```python
from build123d import *

# Parameters (mm, degrees)
F0_R     = 2.5
F1_DEPTH = 25


with BuildPart() as f1:
    # F0 (on Top) → F1 (new body)
    with BuildSketch(Plane.XY):
        with BuildLine():
            Line((-0.206975, 3.902523), (-2.845819, 3.902523))
            Line((-2.845819, 3.902523), (-5.497237, 6.55394))
            Line((-5.497237, 6.55394), (-5.497237, 8.202523))
            Line((-5.497237, 8.202523), (-2.885113, 8.202523))
            Line((-2.885113, 8.202523), (-2.885113, 8.30915))
            Line((-2.885113, 8.30915), (-4.400227, 9.824264))
            ThreePointArc((-4.400227, 9.824264), (-4.594881, 9.954328), (-4.824491, 10))
            Line((-4.824491, 10), (-8.5, 10))
            ThreePointArc((-8.5, 10), (-9.074025, 9.885819), (-9.56066, 9.56066))
            ThreePointArc((-9.56066, 9.56066), (-9.885819, 9.074025), (-10, 8.5))
            Line((-10, 8.5), (-10, 4.824491))
            ThreePointArc((-10, 4.824491), (-9.954328, 4.594881), (-9.824264, 4.400227))
            Line((-9.824264, 4.400227), (-8.30915, 2.885113))
            Line((-8.30915, 2.885113), (-8.202523, 2.885113))
            Line((-8.202523, 2.885113), (-8.202523, 5.497237))
            Line((-8.202523, 5.497237), (-6.55394, 5.497237))
            Line((-6.55394, 5.497237), (-3.902523, 2.845819))
            Line((-3.902523, 2.845819), (-3.902523, 0.206975))
            Line((-3.902523, 0.206975), (-3.695548, 0))
            Line((-3.695548, 0), (-3.902523, -0.206975))
            Line((-3.902523, -0.206975), (-3.902523, -2.845819))
            Line((-3.902523, -2.845819), (-6.55394, -5.497237))
            Line((-6.55394, -5.497237), (-8.202523, -5.497237))
            Line((-8.202523, -5.497237), (-8.202523, -2.885113))
            Line((-8.202523, -2.885113), (-8.30915, -2.885113))
            Line((-8.30915, -2.885113), (-9.824264, -4.400227))
            ThreePointArc((-9.824264, -4.400227), (-9.954328, -4.594881), (-10, -4.824491))
            Line((-10, -4.824491), (-10, -8.5))
            ThreePointArc((-10, -8.5), (-9.885819, -9.074025), (-9.56066, -9.56066))
            ThreePointArc((-9.56066, -9.56066), (-9.074025, -9.885819), (-8.5, -10))
            Line((-8.5, -10), (-4.824491, -10))
            ThreePointArc((-4.824491, -10), (-4.594881, -9.954328), (-4.400227, -9.824264))
            Line((-4.400227, -9.824264), (-2.885113, -8.30915))
            Line((-2.885113, -8.30915), (-2.885113, -8.202523))
            Line((-2.885113, -8.202523), (-5.497237, -8.202523))
            Line((-5.497237, -8.202523), (-5.497237, -6.55394))
            Line((-5.497237, -6.55394), (-2.845819, -3.902523))
            Line((-2.845819, -3.902523), (-0.206975, -3.902523))
            Line((-0.206975, -3.902523), (0, -3.695548))
            Line((0, -3.695548), (0.206975, -3.902523))
            Line((0.206975, -3.902523), (2.845819, -3.902523))
            Line((2.845819, -3.902523), (5.497237, -6.55394))
            Line((5.497237, -6.55394), (5.497237, -8.202523))
            Line((5.497237, -8.202523), (2.885113, -8.202523))
            Line((2.885113, -8.202523), (2.885113, -8.30915))
            Line((2.885113, -8.30915), (4.400227, -9.824264))
            ThreePointArc((4.400227, -9.824264), (4.594881, -9.954328), (4.824491, -10))
            Line((4.824491, -10), (8.5, -10))
            ThreePointArc((8.5, -10), (9.074025, -9.885819), (9.56066, -9.56066))
            ThreePointArc((9.56066, -9.56066), (9.885819, -9.074025), (10, -8.5))
            Line((10, -8.5), (10, -4.824491))
            ThreePointArc((10, -4.824491), (9.954328, -4.594881), (9.824264, -4.400227))
            Line((9.824264, -4.400227), (8.30915, -2.885113))
            Line((8.30915, -2.885113), (8.202523, -2.885113))
            Line((8.202523, -2.885113), (8.202523, -5.497237))
            Line((8.202523, -5.497237), (6.55394, -5.497237))
            Line((6.55394, -5.497237), (3.902523, -2.845819))
            Line((3.902523, -2.845819), (3.902523, -0.206975))
            Line((3.902523, -0.206975), (3.695548, 0))
            Line((3.695548, 0), (3.902523, 0.206975))
            Line((3.902523, 0.206975), (3.902523, 2.845819))
            Line((3.902523, 2.845819), (6.55394, 5.497237))
            Line((6.55394, 5.497237), (8.202523, 5.497237))
            Line((8.202523, 5.497237), (8.202523, 2.885113))
            Line((8.202523, 2.885113), (8.30915, 2.885113))
            Line((8.30915, 2.885113), (9.824264, 4.400227))
            ThreePointArc((9.824264, 4.400227), (9.954328, 4.594881), (10, 4.824491))
            Line((10, 4.824491), (10, 8.5))
            ThreePointArc((10, 8.5), (9.885819, 9.074025), (9.56066, 9.56066))
            ThreePointArc((9.56066, 9.56066), (9.074025, 9.885819), (8.5, 10))
            Line((8.5, 10), (4.824491, 10))
            ThreePointArc((4.824491, 10), (4.594881, 9.954328), (4.400227, 9.824264))
            Line((4.400227, 9.824264), (2.885113, 8.30915))
            Line((2.885113, 8.30915), (2.885113, 8.202523))
            Line((2.885113, 8.202523), (5.497237, 8.202523))
            Line((5.497237, 8.202523), (5.497237, 6.55394))
            Line((5.497237, 6.55394), (2.845819, 3.902523))
            Line((2.845819, 3.902523), (0.206975, 3.902523))
            Line((0.206975, 3.902523), (0, 3.695548))
            Line((0, 3.695548), (-0.206975, 3.902523))
        make_face()
        Polygon((-7.11684, -7.11684), (-6.573574, -7.660106), (-6.573574, -8.202523), (-8.202523, -8.202523), (-8.202523, -6.573574), (-7.660106, -6.573574), align=None, mode=Mode.SUBTRACT)
        Polygon((7.11684, -7.11684), (7.660106, -6.573574), (8.202523, -6.573574), (8.202523, -8.202523), (6.573574, -8.202523), (6.573574, -7.660106), align=None, mode=Mode.SUBTRACT)
        Polygon((-6.573574, 8.202523), (-6.573574, 7.660106), (-7.11684, 7.11684), (-7.660106, 6.573574), (-8.202523, 6.573574), (-8.202523, 8.202523), align=None, mode=Mode.SUBTRACT)
        Circle(F0_R, mode=Mode.SUBTRACT)
        Polygon((7.11684, 7.11684), (6.573574, 7.660106), (6.573574, 8.202523), (8.202523, 8.202523), (8.202523, 6.573574), (7.660106, 6.573574), align=None, mode=Mode.SUBTRACT)
    extrude(amount=F1_DEPTH)


solid = f1.part
```
Input: part model. Units: mm. Frame: model coordinates. A direction names the side the tool comes from. Round coordinates to 2 decimals unless told otherwise and drop trailing zeros. Loops run counter-clockwise (first coordinate to the right, second up) from the corner with the lowest first, then second, coordinate; pieces in that order, holes last. Notation, with made-up numbers: (41, -9.75) - (86, -9.75) arc R32 ccw to (86, 17.25) - close; hole circle Ø4 at (-11, 52.5). An arc over 180 degrees is marked (long way). One line per item, written item: value. Start each with the question number.
(1) Draft query along X for faces 1 (the flat face through (-5.497, -7, 12)), 2 (the flat face through (5.247, -4.19, 12.325)), 3 (the flat face through (-9.056, -3.632, 12.325)). Return one class per face: +X half, -X half, draft (parallel to the pull), parting line (faces both ways), or undercut.
(2) Section A-A, the plane y = 1.5. Return loops of the section in (x, z), plus the area to 3 significant figures.
(3) Access query for faces 4 (the flat face through (-7, -8.203, 12)), 5 (the flat face through (2, -3.903, 12)). Directions: +Z, -Z, +X, -X, +Y, -Y. A direction counts if a zero-diameter tool reaches every point of the face in a straight line with its end or side. Return the directions, or none.
(4) Section C-C, the plane z = 16.25. Count the separate pieces of the cut face and the enclosed holes in it, plus the area to 3 significant figures.
(5) Ray query, line 1 (X direction, y = -3, z = 10.75); line 2 (Y direction, x = -5, z = 16); line 3 (Y direction, x = -2.75, z = 13.5). Return the intervals inside material, ascending. Write a range as [from, to].
(6) Contact query for flat-ended pins moving along their axis: P1, Ø1, axis at x = -2.5, z = 8.5, coming from the +Y side; P2, Ø0.8, axis at y = 1, z = 8, coming from the +X side; P3, Ø0.8, axis at y = 1.5, z = 6.5, coming from the -X side; P4, Ø1.5, axis at x = 6.5, y = -1.5, coming from the -Z side. Output: stop coordinate, or through.
(7) Section B-B, the plane x = 6.25. Return loops of the section in (y, z).
Results below:
1. face 1: undercut
1. face 2: undercut
1. face 3: -X half
2. outline: (-3.9, 0) - (-2, 0) - (-2, 25) - (-3.9, 25) - close; (2, 0) - (3.9, 0) - (3.9, 25) - (2, 25) - close
2. area: 95.1 mm^2
3. face 4: +Z, -Z
3. face 5: +Z, -Z, -Y
4. separate pieces: 1
4. enclosed holes: 5
4. area: 156 mm^2
5. line 1: [-8.42, -8.2], [-4.06, 4.06], [8.2, 8.42]
5. line 2: [-10, -8.2], [-6.06, -3.94], [3.94, 6.06], [8.2, 10]
5. line 3: [-3.9, 3.9]
6. P1: y = 8.42
6. P2: x = 3.9
6. P3: x = -3.9
6. P4: through
7. outline: (-10, 0) - (-5.19, 0) - (-5.19, 25) - (-10, 25) - close; (5.19, 0) - (10, 0) - (10, 25) - (5.19, 25) - close
